Geometry check sheet. Reference: the model listing, model coordinates, mm. Face numbers are marked on the shaded views. Round coordinates to 2 decimals unless told otherwise and drop trailing zeros. Order: outer loops, then holes, each group sorted by start corner. A loop starts at its lowest first (then second) coordinate and runs counter-clockwise, first axis right, second up.
```python
from build123d import *

# Parameters (mm, degrees)
F0_R      = 10
F0_R_2    = 6
F1_DEPTH  = 50
F2_R      = 10
F3_DEPTH  = 5
F4_R      = 8.0824379909
F5_DEPTH  = 15
F6_R      = 2.5
F7_DEPTH  = 55.001
F8_SIZE   = 1
F11_D     = 4.2
F11_DEPTH = 7.4
F11_START = 0.2229862
F11_TIP   = 1.2618073


with BuildPart() as f1:
    # F0 (on Front) → F1 (new body)
    with BuildSketch(Plane.XZ):
        Circle(F0_R)
        Circle(F0_R_2, mode=Mode.SUBTRACT)
    extrude(amount=F1_DEPTH)

    # F2 (on face) → F3 (join)
    with BuildSketch(Plane(origin=(0, 0, 0), x_dir=(-1, 0, 0), z_dir=(0, 1, 0))):
        Circle(F2_R)
    extrude(amount=F3_DEPTH)

    # F4 (on face) → F5 (cut)
    with BuildSketch(Plane.XZ.offset(50)):
        Circle(F4_R)
    extrude(amount=-F5_DEPTH, mode=Mode.SUBTRACT)

    # F6 (on face) → F7 (cut, through all)
    with BuildSketch(Plane(origin=(0, 5, 0), x_dir=(-1, 0, 0), z_dir=(0, 1, 0))):
        Circle(F6_R)
    extrude(amount=-F7_DEPTH, mode=Mode.SUBTRACT)

    # F8
    f8_edges = [f1.edges().sort_by_distance(p)[0] for p in [
        (10, 5, 0),
    ]]
    chamfer(f8_edges, length=F8_SIZE)

    # F11
    # its depths count from where the whole tool has entered the part; down to there all is cleared
    with Locations(Plane.YZ.offset(10).offset(-F11_START)):
        with Locations((-25, 0), (-3, 0)):
            Hole(F11_D / 2, depth=F11_DEPTH)
            with Locations((0, 0, -(F11_DEPTH + F11_TIP / 2))):  # 118° drill point
                Cone(0, F11_D / 2, F11_TIP, mode=Mode.SUBTRACT)


solid = f1.part
```
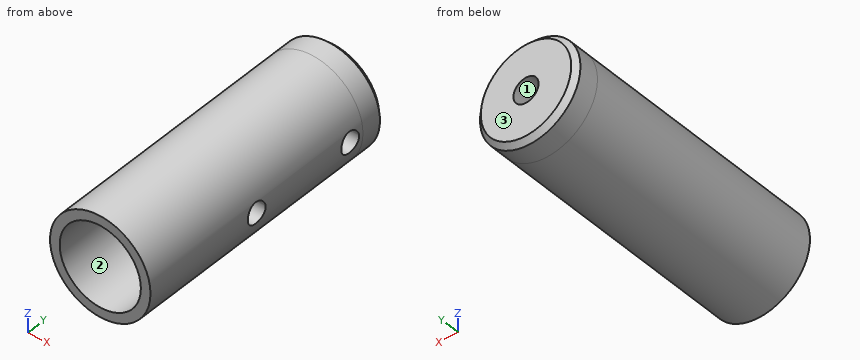
(1) Sectioned sample at A-A, the plane z = 0. Record the cut outline in (x, y), and give its area (3 significant figures).
Returned:
outline: (-10, -50) - (-8.08, -50) - (-8.08, -35) - (-6, -35) - (-6, 0) - (-2.5, 0) - (-2.5, 5) - (-9, 5) - (-10, 4) - close; (2.5, 0) - (6, 0) - (6, -0.9) - (10, -0.9) - (10, 4) - (9, 5) - (2.5, 5) - close; (6, -35) - (8.08, -35) - (8.08, -50) - (10, -50) - (10, -27.1) - (6, -27.1) - close; (6, -22.9) - (10, -22.9) - (10, -5.1) - (6, -5.1) - close
area: 378 mm2
(2) Material ranges on line 1 (Z direction, x = 0, y = 1.1); line 2 (Z direction, x = 0, y = -9.5); line 3 (X direction, y = -42.5, z = -2), recorded low to high.
Returned:
line 1: z = -10 to -2.5, 2.5 to 10
line 2: z = -10 to -6, 6 to 10
line 3: x = -9.8 to -7.83, 7.83 to 9.8
(3) Sectioned sample at D-D, the plane y = -25. Record the cut outline in (x, z).
Returned:
outline: (5.62, -2.1) arc R6 cw (long way) to (5.62, 2.1) - (9.78, 2.1) arc R10 ccw (long way) to (9.78, -2.1) - close
(4) Draft check along Z on the marked faces 1, 2 and 3. Enter one of: released by +Z, released by -Z, zero draft, split by the parting line, or undercut.
Returned:
face 1: undercut
face 2: undercut
face 3: zero draft
(5) Sectioned sample at B-B, the plane x = 0. Record the cut outline in (y, z).
Returned:
outline: (-50, -10) - (4, -10) - (5, -9) - (5, -2.5) - (0, -2.5) - (0, -6) - (-35, -6) - (-35, -8.08) - (-50, -8.08) - close; (-50, 8.08) - (-35, 8.08) - (-35, 6) - (0, 6) - (0, 2.5) - (5, 2.5) - (5, 9) - (4, 10) - (-50, 10) - close
(6) Sectioned sample at C-C, the plane y = -35.5. Record the cut outline in (x, z), and give its area (3 significant figures).
Returned:
outline: circle Ø20 at (0, 0); hole circle Ø16.16 at (0, 0)
area: 109 mm2
(7) Depth check by flat-ended pin: P1, Ø8, axis at x = -4.5, y = -41, coming from the -Z side; P2, Ø5, axis at y = -12, z = -4, coming from the +X side; P3, Ø8, axis at x = 0, z = 0, coming from the +Y side; P4, Ø1, axis at x = -5.5, y = -33, coming from the +Z side. Enter the tip coordinate at first touch or a pass-through.
Returned:
P1: stops at z = -9.99
P2: stops at x = 9.89
P3: stops at y = 5
P4: stops at z = 8.66
